```python
from build123d import *

# Parameters (mm, degrees)
SKETCH1_W           = 116
SKETCH1_H           = 62
BOSS_EXTRUDE1_DEPTH = 2
SKETCH2_R           = 1.75
CUT_EXTRUDE1_DEPTH  = 2
SKETCH3_R           = 1.75
CUT_EXTRUDE2_DEPTH  = 2
FILLET2_R           = 10


with BuildPart() as part:
    # Sketch1 → Boss-Extrude1 (new body)
    with BuildSketch(Plane(origin=(0, 0, 0), x_dir=(1, 0, 0), z_dir=(0, 1, 0))):
        Rectangle(SKETCH1_W, SKETCH1_H)
    extrude(amount=BOSS_EXTRUDE1_DEPTH)

    # Sketch2 → Cut-Extrude1 (cut)
    with BuildSketch(Plane(origin=(0, 2, 0), x_dir=(1, 0, 0), z_dir=(0, 1, 0))):
        with Locations(Location((-48, 27, 0), (0, 0, 270))):
            Circle(SKETCH2_R)
        with Locations(Location((48, 27, 0), (0, 0, 270))):
            Circle(SKETCH2_R)
        with Locations(Location((48, -27, 0), (0, 0, 270))):
            Circle(SKETCH2_R)
        with Locations(Location((-48, -27, 0), (0, 0, 270))):
            Circle(SKETCH2_R)
    extrude(amount=-CUT_EXTRUDE1_DEPTH, mode=Mode.SUBTRACT)

    # Sketch3 → Cut-Extrude2 (cut)
    with BuildSketch(Plane(origin=(0, 2, 0), x_dir=(1, 0, 0), z_dir=(0, 1, 0))):
        with Locations(Location((25, 0, 0), (0, 0, 270))):
            Circle(SKETCH3_R)
        with Locations(Location((-25, 0, 0), (0, 0, 270))):
            Circle(SKETCH3_R)
        with BuildLine():
            Line((9.5, -19), (29.5, -19))
            ThreePointArc((29.5, -19), (31, -20.5), (29.5, -22))
            Line((29.5, -22), (9.5, -22))
            ThreePointArc((9.5, -22), (8, -20.5), (9.5, -19))
        make_face()
        with BuildLine():
            Line((-9.5, -22), (-29.5, -22))
            ThreePointArc((-29.5, -22), (-31, -20.5), (-29.5, -19))
            Line((-29.5, -19), (-9.5, -19))
            ThreePointArc((-9.5, -19), (-8, -20.5), (-9.5, -22))
        make_face()
        with BuildLine():
            Line((-29.5, 22), (-9.5, 22))
            ThreePointArc((-9.5, 22), (-8, 20.5), (-9.5, 19))
            Line((-9.5, 19), (-29.5, 19))
            ThreePointArc((-29.5, 19), (-31, 20.5), (-29.5, 22))
        make_face()
        with BuildLine():
            Line((9.5, 22), (29.5, 22))
            ThreePointArc((29.5, 22), (31, 20.5), (29.5, 19))
            Line((29.5, 19), (9.5, 19))
            ThreePointArc((9.5, 19), (8, 20.5), (9.5, 22))
        make_face()
        Polygon((-35.6, 12.5), (-39.2, 18.735382907), (-46.4, 18.735382907), (-50, 12.5), (-46.4, 6.264617093), (-39.2, 6.264617093), align=None)
        Polygon((-35.6, -12.5), (-39.2, -6.264617093), (-46.4, -6.264617093), (-50, -12.5), (-46.4, -18.735382907), (-39.2, -18.735382907), align=None)
        Polygon((50, 12.5), (46.4, 18.735382907), (39.2, 18.735382907), (35.6, 12.5), (39.2, 6.264617093), (46.4, 6.264617093), align=None)
        Polygon((50, -12.5), (46.4, -6.264617093), (39.2, -6.264617093), (35.6, -12.5), (39.2, -18.735382907), (46.4, -18.735382907), align=None)
    extrude(amount=-CUT_EXTRUDE2_DEPTH, mode=Mode.SUBTRACT)

    # Fillet2
    fillet2_edges = [part.edges().sort_by_distance(p)[0] for p in [
        (58, 1, 31),
        (-58, 1, 31),
        (-58, 1, -31),
        (58, 1, -31),
    ]]
    fillet(fillet2_edges, radius=FILLET2_R)


solid = part.part
```
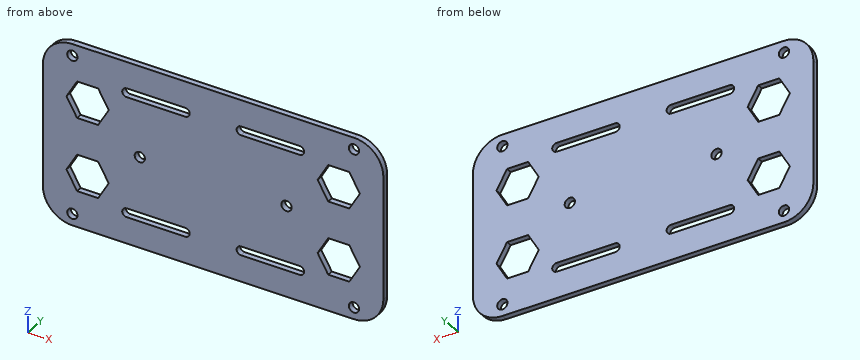
Could you check a few things on this model? Use its own coordinates, in mm. Coordinates: 2 decimals unless noted, no trailing zeros. Write each loop counter-clockwise with the first axis right and the second up, starting at its lowest first coordinate (ties: lowest second). Pieces come first, ordered by that corner, then holes. Notation, with made-up numbers: (-1.75, 69.5) -> (38.25, 69.5) arc R35 ccw to (38.25, 102.5) -> close; hole circle Ø11 at (14.25, 39). An arc over 180 degrees is marked (long way). Return JSON: item names as keys, results as strings.
(1) Imagine slicing it at A-A, the plane z = 0. Please give me the cut outline in (x, y).
Numbers:
{"outline": "(-58, 0) -> (-26.75, 0) -> (-26.75, 2) -> (-58, 2) -> close; (-23.25, 0) -> (23.25, 0) -> (23.25, 2) -> (-23.25, 2) -> close; (26.75, 0) -> (58, 0) -> (58, 2) -> (26.75, 2) -> close"}
(2) I'm going to push a flat-ended pin straight in: pin 1 (3 mm diameter, centred on x = 48, z = 27, fed in from -Y). Where does the tip first touch, or does it pass through?
Numbers:
{"pin 1": "passes through"}
(3) I need wall thicknesses on L1, parallel to Z at x = 21, y = 0.3; L2, parallel to X at y = 1.5, z = 0; L3, parallel to Z at x = 39, y = 0.6. Which ranges of each line are inside material? Lowest first, please.
Numbers:
{"L1": "z = -31 to -22, -19 to 19, 22 to 31", "L2": "x = -58 to -26.75, -23.25 to 23.25, 26.75 to 58", "L3": "z = -31 to -18.39, -6.61 to 6.61, 18.39 to 31"}
(4) Imagine slicing it at B-B, the plane x = -12. Please give me the cut outline in (y, z).
Numbers:
{"outline": "(0, -31) -> (2, -31) -> (2, -22) -> (0, -22) -> close; (0, -19) -> (2, -19) -> (2, 19) -> (0, 19) -> close; (0, 22) -> (2, 22) -> (2, 31) -> (0, 31) -> close"}
(5) Imagine slicing it at D-D, the plane y = 1. Count the separate pieces of the cut face and the enclosed holes in it, then the cut area to 3 significant figures.
Numbers:
{"separate pieces": "1", "enclosed holes": "14", "area": "6,240 mm2"}
(6) Imagine slicing it at C-C, the plane x = 25. Please give me the cut outline in (y, z).
Numbers:
{"outline": "(0, -31) -> (2, -31) -> (2, -22) -> (0, -22) -> close; (0, -19) -> (2, -19) -> (2, -1.75) -> (0, -1.75) -> close; (0, 1.75) -> (2, 1.75) -> (2, 19) -> (0, 19) -> close; (0, 22) -> (2, 22) -> (2, 31) -> (0, 31) -> close"}
